Work out the finished part from the listing and answer in its coordinate system (mm). A direction names the side the tool comes from. Round coordinates to 2 decimals unless told otherwise and drop trailing zeros. Order: outer loops, then holes, each group sorted by start corner. A loop starts at its lowest first (then second) coordinate and runs counter-clockwise, first axis right, second up. Notation, with made-up numbers: (20.25, 79.5) - (67.25, 79.5) arc R31 ccw to (67.25, 117.5) - close; hole circle Ø3 at (69.25, 88). An arc over 180 degrees is marked (long way). Put each result on its own line as item: value.
```python
from build123d import *

# Parameters (mm, degrees)
CHAMFER_2_SIZE           = 2
SKETCH_6_W               = 3
SKETCH_6_H               = 4
SKETCH_7_W               = 10
SKETCH_7_H               = 3.436723268
EXTRUDE_1_DEPTH          = 1.5
PATTERN_CIRCULAR_1_COUNT = 20


with BuildPart() as part:
    # Эскиз4 → Повернуть1 (revolve)
    with BuildSketch(Plane.XY, mode=Mode.PRIVATE) as revolve_1_sk:
        Polygon((0, 22.5), (-30, 22.5), (-30, 18.5), (-19, 18.5), (-19, 5.1), (-13, 5.1), (-13, 3.15), (-6.2, 3.15), (-6.2, 9.7), (0, 9.7), align=None)
    revolve(revolve_1_sk.sketch.rotate(Axis((-30, 0, 0), (1, 0, 0)), 90), axis=Axis((-30, 0, 0), (1, 0, 0)))

    # Фаска2
    chamfer_2_edges = [part.edges().sort_by_distance(p)[0] for p in [
        (-19, 0, -18.5),
        (-30, 0, -18.5),
    ]]
    chamfer(chamfer_2_edges, length=CHAMFER_2_SIZE)

    # Эскиз6 → Вырез-Повернуть2 (revolve, cut)
    with BuildSketch(Plane.XY, mode=Mode.PRIVATE) as cut_revolve_2_sk:
        with Locations((-24.5, 21.5)):
            Rectangle(SKETCH_6_W, SKETCH_6_H)
        with Locations((-5.5, 21.5)):
            Rectangle(SKETCH_6_W, SKETCH_6_H)
    revolve(cut_revolve_2_sk.sketch.rotate(Axis((-30, 0, 0), (1, 0, 0)), 90), axis=Axis((-30, 0, 0), (1, 0, 0)), mode=Mode.SUBTRACT)

    # Эскиз7 → Бобышка-Вытянуть1 (add, symmetric)
    with BuildSketch(Plane.XY):
        with Locations((-15, 22.781638366)):
            Rectangle(SKETCH_7_W, SKETCH_7_H)
    extrude_1 = extrude(amount=EXTRUDE_1_DEPTH, both=True)

    # Круговой массив1: Бобышка-Вытянуть1 ×20 about axis
    pattern_circular_1_axis = Axis((0, 0, 0), (1, 0, 0))
    for i in range(1, PATTERN_CIRCULAR_1_COUNT):
        add(extrude_1.rotate(pattern_circular_1_axis, i * 360 / PATTERN_CIRCULAR_1_COUNT))


solid = part.part
```
1) Given pin 1 Ø0.6 at (x, z) = (-13, 23) entering from -Y; pin 2 Ø3 at (x, y) = (-13.5, -3.5) entering from -Z; pin 3 Ø9 at (y, z) = (0, 0) entering from -X, each flat-ended and moving along its own axis, determine where each tip first touches the part or whether it passes through.
Findings below:
pin 1: stops at y = -9
pin 2: stops at z = -22.41
pin 3: stops at x = -13
2) For a pull along Y with two mould halves and no side action, classify faces 1 (the flat face through (-15.07, -23.307, 7.551)), 2 (the flat face through (-15.07, 8.685, -21.876)), 3 (the flat face through (-20, -7, -22)), 4 (the cylindrical face through (-24.45, 16.41, 8.54)) as pulls with the +Y half, pulls with the -Y half, needs draft (parallel to the pull), parting line crosses it, or undercut.
Findings below:
face 1: pulls with the -Y half
face 2: pulls with the +Y half
face 3: needs draft
face 4: undercut
3) A cutting plane is placed at A-A on x = -22.25. Write down the section's boundary in (y, z).
Findings below:
outline: circle Ø45 at (0, 0); hole circle Ø37 at (0, 0)
4) Straight lines are drawn through the part: L1, parallel to X at y = -20.5, z = -7; L2, parallel to Y at x = -23.5, z = 0; L3, parallel to Y at x = -8.5, z = 0. For each, find the intervals that lie inside material, in ascending order. Write a range as from..to.
Findings below:
L1: x = -30..-26, -23..-7, -4..0
L2: y = -19.5..-18.5, 18.5..19.5
L3: y = -22.5..-3.15, 3.15..22.5
5) For faces 5 (the flat face through (-10, -19, 14)), 6 (the cylindrical face through (-2.028, 19.961, 10.382)), 7 (the flat face through (-15, -23, 1.5)), 8 (the flat face through (-20, 14, 19)), 9 (the flat face through (-13, -0.1, 3.3)), determine the directions among +Z, -Z, +X, -X, +Y, -Y from which every point of the face is accessible in a straight line to the end or side of a thin tool.
Findings below:
face 5: +Z, +X, -Y
face 6: +X
face 7: +X, -X, -Y
face 8: +Z, -X, +Y
face 9: -X
